For this review, take the finished solid that the model builds, in its own axes (mm). A direction names the side the tool comes from. Coordinates: 2 decimals unless noted, no trailing zeros. Loops run counter-clockwise (first coordinate to the right, second up) from the corner with the lowest first, then second, coordinate; pieces in that order, holes last. Notation, with made-up numbers: (85, 30) - (139, 30) arc R10 cw to (139, 47) - close; hole circle Ø11 at (-14, 31). An arc over 180 degrees is marked (long way). Use one line per item in the form item = value. Start each with the question number.
1. Machinability: for faces 1 (the face through (-7, 0, -2)), 2 (the face through (3, 0, -1)), 3 (the face through (4, 0, -2)), which of the approach directions +Z, -Z, +X, -X, +Y, -Y give a long, thin tool a straight path to every point of the face, cutting with its end or side? Answer none if there is none.
2. Add section C-C on x = -1. Give the boundary of the cut face in (y, z).
3. Add section A-A on y = 0. Give the boundary of the cut face in (x, z).
4. Add section D-D on x = 1.5. Give the boundary of the cut face in (y, z).
5. To check wall thickness, follow probe 1 along X at (y, z) = (0.25, 2.25); probe 2 along X at (y, z) = (0.75, -0.75); probe 3 along Z at (x, y) = (-5.25, -1). State the ranges of each line that lie inside material, in increasing order.
6. Add section B-B on z = 0. Give the boundary of the cut face in (x, y), and give its area (3 significant figures).
7. For pin 1 Ø2 at (x, y) = (3.5, 2) entering from +Z; pin 2 Ø1.5 at (x, y) = (-10, -2.5) entering from -Z; pin 3 Ø3 at (x, z) = (-3, 2) entering from -Y, all flat-tipped, find the tip position at first contact; note any pin that passes through.
Autodesk Inventor part; units mm, degrees
ref_plane "YZ Plane" through (0, 0, 0) normal (1, 0, 0) x (0, 1, 0)
ref_plane "XZ Plane" through (0, 0, 0) normal (0, 1, 0) x (-1, 0, 0)
ref_plane "XY Plane" through (0, 0, 0) normal (0, 0, 1) x (1, 0, 0)
sketch "Sketch1" plane through (0, 0, 0) normal (1, 0, 0) x (0, 1, 0)
  circle A0 centre (0, 0) radius 2
  circle A1 centre (0, 0) radius 3.75
  dimension "d0" = 4
  dimension "d1" = 7.5
extrude "Extrusion1" add sketch "Sketch1" against normal blind 16 contours A0
extrude "Extrusion2" add sketch "Sketch1" along normal blind 4 contours A0 | A1
sketch "Sketch2" plane through (4, 0, 0) normal (1, 0, 0) x (0, 0, -1)
  circle A0 centre (0, 0) radius 3.75
  circle A1 centre (0, 0) radius 3.75
  line L0 (-1, -3.6142) -> (-1, 3.6142)
  line L1 (1, -3.6142) -> (1, 3.6142)
  line L2 (0, 0) -> (0, 3.75)
  dimension "d15" = 2
extrude "Extrusion3" cut sketch "Sketch2" against normal blind 2 contours L1 A0 L0
chamfer "Chamfer1" distance 0.8 angle 45 1 edges at (-16, -2, 0)
thread "Thread2"
properties part number "screw_M3-10" material "Сталь"
Conclusion:
q1.face_1 = -X
q1.face_2 = +X, +Y, -Y
q1.face_3 = +Z, -Z, +X, +Y, -Y
q2.outline = circle Ø4 at (0, 0)
q3.outline = (-16, -1.2) - (-15.2, -2) - (0, -2) - (0, -3.75) - (4, -3.75) - (4, -1) - (2, -1) - (2, 1) - (4, 1) - (4, 3.75) - (0, 3.75) - (0, 2) - (-15.2, 2) - (-16, 1.2) - close
q4.outline = circle Ø7.5 at (0, 0)
q5.probe_1 = 0 to 4
q5.probe_2 = -16 to 2
q5.probe_3 = -1.73 to 1.73
q6.outline = (-16, -1.2) - (-15.2, -2) - (0, -2) - (0, -3.75) - (2, -3.75) - (2, 3.75) - (0, 3.75) - (0, 2) - (-15.2, 2) - (-16, 1.2) - close
q6.area = 78.4 mm^2
q7.pin_1 = 3.61
q7.pin_2 = -0.97
q7.pin_3 = -1.94
